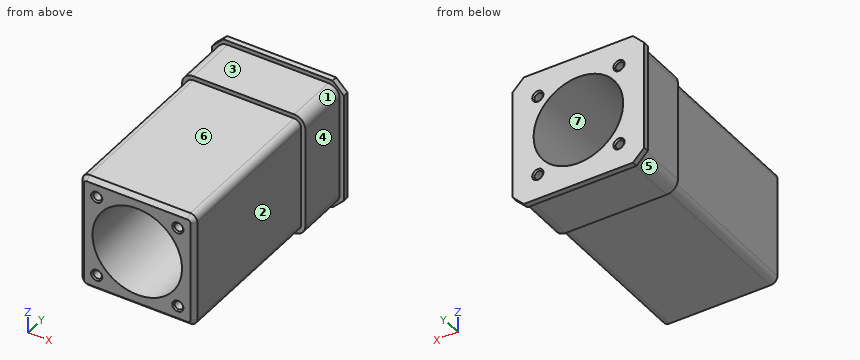
```python
from build123d import *

# Parameters (mm, degrees)
SKETCH_1_W                    = 41
SKETCH_1_H                    = 41
EXTRUDE_1_DEPTH               = 59
SKETCH_2_W                    = 44
SKETCH_2_H                    = 44
EXTRUDE_2_DEPTH               = 19
SKETCH_3_W                    = 47
SKETCH_3_H                    = 47
EXTRUDE_3_DEPTH               = 2
FILLET_1_R                    = 2.5
FILLET_2_R                    = 4
CHAMFER_1_SIZE                = 1.5
CHAMFER_2_SIZE                = 4
SKETCH_4_R                    = 16
CUT_EXTRUDE_4_DEPTH           = 81
M4X0_71_D                     = 3
M4X0_71_DEPTH                 = 14
M4X0_71_CSINK_D               = 4
M4X0_71_CSINK_ANGLE           = 90
M4X0_71_TIP                   = 0.901290929
M4X0_71_ON_FACE_2_D           = 3
M4X0_71_ON_FACE_2_DEPTH       = 14
M4X0_71_ON_FACE_2_CSINK_D     = 4
M4X0_71_ON_FACE_2_CSINK_ANGLE = 90
M4X0_71_ON_FACE_2_TIP         = 0.901290929


with BuildPart() as part:
    # Эскиз1 → Вытянуть1 (new body)
    with BuildSketch(Plane(origin=(0, 0, 0), x_dir=(1, 0, 0), z_dir=(0, 1, 0))):
        Rectangle(SKETCH_1_W, SKETCH_1_H)
    extrude(amount=EXTRUDE_1_DEPTH)

    # Эскиз2 → Вытянуть2 (add)
    with BuildSketch(Plane(origin=(0, 59, 0), x_dir=(1, 0, 0), z_dir=(0, 1, 0))):
        Rectangle(SKETCH_2_W, SKETCH_2_H)
    extrude(amount=EXTRUDE_2_DEPTH)

    # Эскиз3 → Вытянуть3 (add)
    with BuildSketch(Plane(origin=(0, 78, 0), x_dir=(1, 0, 0), z_dir=(0, 1, 0))):
        Rectangle(SKETCH_3_W, SKETCH_3_H)
    extrude(amount=EXTRUDE_3_DEPTH)

    # Скругление1
    fillet_1_edges = [part.edges().sort_by_distance(p)[0] for p in [
        (20.5, 29.5, 20.5),
        (-20.5, 29.5, 20.5),
        (-20.5, 29.5, -20.5),
        (20.5, 29.5, -20.5),
    ]]
    fillet(fillet_1_edges, radius=FILLET_1_R)

    # Скругление2
    fillet_2_edges = [part.edges().sort_by_distance(p)[0] for p in [
        (22, 68.5, 22),
        (22, 68.5, -22),
        (-22, 68.5, -22),
        (-22, 68.5, 22),
    ]]
    fillet(fillet_2_edges, radius=FILLET_2_R)

    # Фаска1
    chamfer_1_edges = [part.edges().sort_by_distance(p)[0] for p in [
        (-20.5, 0, 0),
        (20.5, 0, 0),
        (0, 0, 20.5),
        (0, 0, -20.5),
        (19.767766953, 0, 19.767766953),
        (19.767766953, 0, -19.767766953),
        (-19.767766953, 0, 19.767766953),
        (-19.767766953, 0, -19.767766953),
    ]]
    chamfer(chamfer_1_edges, length=CHAMFER_1_SIZE)

    # Фаска2
    chamfer_2_edges = [part.edges().sort_by_distance(p)[0] for p in [
        (23.5, 79, 23.5),
        (23.5, 79, -23.5),
        (-23.5, 79, -23.5),
        (-23.5, 79, 23.5),
    ]]
    chamfer(chamfer_2_edges, length=CHAMFER_2_SIZE)

    # Эскиз4 → Вытянуть4 (cut, through all)
    with BuildSketch(Plane(origin=(0, 80, 0), x_dir=(1, 0, 0), z_dir=(0, 1, 0))):
        Circle(SKETCH_4_R)
    extrude(amount=-CUT_EXTRUDE_4_DEPTH, mode=Mode.SUBTRACT)

    # Отверстие обработанное метчиком M4x0.71
    with Locations(Plane(origin=(-14.495689014, 0, 14.495689014), x_dir=(0, 0, -1), z_dir=(0, -1, 0))):
        with Locations((0, 0), (28.991378028, 0), (28.991378028, 28.991378028), (0, 28.991378028)):
            CounterSinkHole(M4X0_71_D / 2, M4X0_71_CSINK_D / 2, depth=M4X0_71_DEPTH, counter_sink_angle=M4X0_71_CSINK_ANGLE)
            with Locations((0, 0, -(M4X0_71_DEPTH + M4X0_71_TIP / 2))):  # 118° drill point
                Cone(0, M4X0_71_D / 2, M4X0_71_TIP, mode=Mode.SUBTRACT)

    # Отверстие обработанное метчиком M4x0.71 on face 2
    with Locations(Plane(origin=(-14.495689014, 80, 14.495689014), x_dir=(0, 0, 1), z_dir=(0, 1, 0))):
        with Locations((0, 0), (0, 28.991378028), (-28.991378028, 28.991378028), (-28.991378028, 0)):
            CounterSinkHole(M4X0_71_ON_FACE_2_D / 2, M4X0_71_ON_FACE_2_CSINK_D / 2, depth=M4X0_71_ON_FACE_2_DEPTH, counter_sink_angle=M4X0_71_ON_FACE_2_CSINK_ANGLE)
            with Locations((0, 0, -(M4X0_71_ON_FACE_2_DEPTH + M4X0_71_ON_FACE_2_TIP / 2))):  # 118° drill point
                Cone(0, M4X0_71_ON_FACE_2_D / 2, M4X0_71_ON_FACE_2_TIP, mode=Mode.SUBTRACT)


solid = part.part
```
For this review, take the finished solid that the model builds, in its own axes (mm). Face numbers are marked on the shaded views. A direction names the side the tool comes from. Coordinates: 2 decimals unless noted, no trailing zeros. Loops run counter-clockwise (first coordinate to the right, second up) from the corner with the lowest first, then second, coordinate; pieces in that order, holes last. Notation, with made-up numbers: (83, 2.25) - (120, 2.25) arc R20 cw to (120, 40.25) - close; hole circle Ø6 at (66.25, 15). An arc over 180 degrees is marked (long way). Use one line per item in the form item = value. Start each with the question number.
1) Take a section at D-D (y = 12). State the section outline as (x, z) points.
2) For pin 1 (6 mm diameter, centred on x = 2, y = 42, fed in from +Z); pin 2 (2.5 mm diameter, centred on x = -14.5, z = -14.5, fed in from +Y); pin 3 (18 mm diameter, centred on y = 17.5, z = -7.5, fed in from -X), all flat-tipped, find the tip position at first contact; note any pin that passes through.
3) Take a section at B-B (x = 0). State the section outline as (y, z) points.
4) For the marked faces 1, 2 and 3, list the 3-axis set-ups (+Z, -Z, +X, -X, +Y, -Y) from which the entire face can be reached by the end or side of a thin tool; tool diameter is ignored.
5) Take a section at C-C (y = 57.5). State the section outline as (x, z) points, plus the area to 3 significant figures.
6) Take a section at A-A (z = 0). State the section outline as (x, y) points, plus the area to 3 significant figures.
7) To check wall thickness, follow probe 1 along X at (y, z) = (19, 0); probe 2 along Z at (x, y) = (8.5, 75); probe 3 along Z at (x, y) = (12, 35). State the ranges of each line that lie inside material, in increasing order. Write a range as from..to.
8) Draft analysis for pull direction X (two halves, no side actions). For the marked faces 4, 5, 6 and 7, state which applies: released by +X, released by -X, zero draft, split by the parting line, or undercut.
From the geometry:
q1.outline = (-20.5, -18) arc R2.5 ccw to (-18, -20.5) - (18, -20.5) arc R2.5 ccw to (20.5, -18) - (20.5, 18) arc R2.5 ccw to (18, 20.5) - (-18, 20.5) arc R2.5 ccw to (-20.5, 18) - close; hole circle Ø3 at (-14.5, -14.5); hole circle Ø32 at (0, 0); hole circle Ø3 at (-14.5, 14.5); hole circle Ø3 at (14.5, -14.5); hole circle Ø3 at (14.5, 14.5)
q2.pin_1 = 20.5
q2.pin_2 = 65.85
q2.pin_3 = -20.5
q3.outline = (0, -19) - (1.5, -20.5) - (59, -20.5) - (59, -22) - (78, -22) - (78, -23.5) - (80, -23.5) - (80, -16) - (0, -16) - close; (0, 16) - (80, 16) - (80, 23.5) - (78, 23.5) - (78, 22) - (59, 22) - (59, 20.5) - (1.5, 20.5) - (0, 19) - close
q4.face_1 = +Z, +X, -Y
q4.face_2 = +Z, -Z, +X, -Y
q4.face_3 = +Z, +X, -X, -Y
q5.outline = (-20.5, -18) arc R2.5 ccw to (-18, -20.5) - (18, -20.5) arc R2.5 ccw to (20.5, -18) - (20.5, 18) arc R2.5 ccw to (18, 20.5) - (-18, 20.5) arc R2.5 ccw to (-20.5, 18) - close; hole circle Ø32 at (0, 0)
q5.area = 871 mm2
q6.outline = (-23.5, 78) - (-22, 78) - (-22, 59) - (-20.5, 59) - (-20.5, 1.5) - (-19, 0) - (-16, 0) - (-16, 80) - (-23.5, 80) - close; (16, 0) - (19, 0) - (20.5, 1.5) - (20.5, 59) - (22, 59) - (22, 78) - (23.5, 78) - (23.5, 80) - (16, 80) - close
q6.area = 787 mm2
q7.probe_1 = -20.5..-16, 16..20.5
q7.probe_2 = -22..-13.56, 13.56..22
q7.probe_3 = -20.5..-10.58, 10.58..20.5
q8.face_4 = released by +X
q8.face_5 = released by -X
q8.face_6 = zero draft
q8.face_7 = undercut
